Autodesk Inventor part; units mm, degrees
ref_plane "YZ Plane" through (0, 0, 0) normal (1, 0, 0) x (0, 1, 0)
ref_plane "XZ Plane" through (0, 0, 0) normal (0, 1, 0) x (-1, 0, 0)
ref_plane "XY Plane" through (0, 0, 0) normal (0, 0, 1) x (1, 0, 0)
sketch "Sketch1" plane through (0, 0, 0) normal (0, 0, 1) x (1, 0, 0)
  circle A0 centre (0, 0) radius 10.1
  circle A1 centre (0, 0) radius 25
  circle A2 centre (0, 0) radius 17.5 construction
  circle A3 centre (0, 17.5) radius 3
  circle A4 centre (-17.5, 0) radius 3
  circle A5 centre (0, -17.5) radius 3
  circle A6 centre (17.5, 0) radius 3
  line L0 (0, 0) -> (0, 17.5)
  line L1 (0, 0) -> (17.5, 0) construction
  dimension "d0" = 20.2
  dimension "d1" = 50
  dimension "d2" = 35
  dimension "d3" = 6
  dimension "d6" = 360
  dimension "d8" = 90
extrude "Extrusion1" add sketch "Sketch1" along normal blind 5
properties part number "JTW20" material "Brass, Soft Yellow"
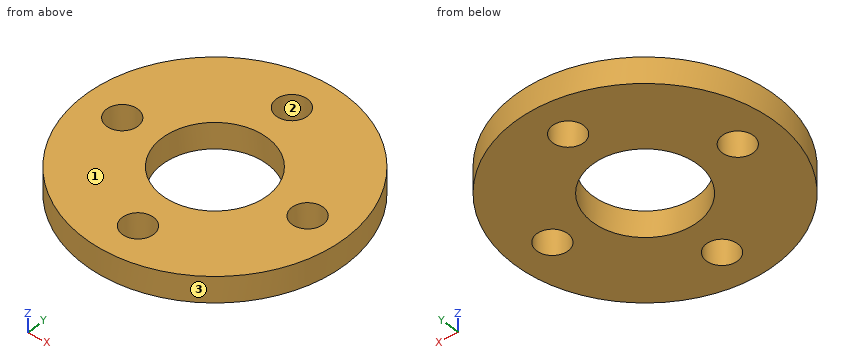
Verification items for the finished model (mm, model axes). Face numbers are marked on the shaded views. Coordinates: 2 decimals unless noted, no trailing zeros. Order: outer loops, then holes, each group sorted by start corner. A loop starts at its lowest first (then second) coordinate and runs counter-clockwise, first axis right, second up. Notation, with made-up numbers: M 16.5,-33 L 73.5,-33 A23 ccw 73.5,-9 Z; hole C -8.75,54 d10. An arc over 180 degrees is marked long. One line per item, written item: value. Start each with the question number.
Item 1: Gauge pin test, flat ends, axial feed: pin 1 (8 mm diameter, centred on x = 0, y = -17.5, fed in from +Z); pin 2 (2 mm diameter, centred on x = 14.5, z = 3.5, fed in from +Y). Record the tip position at first contact, or that the pin passes through.
Item 2: Mould release check, pull along X, two halves, no side actions. Record for the marked faces 1, 2 and 3: released by +X, released by -X, zero draft, split by the parting line, or undercut.
Item 3: Scan lines: probe 1 along Y at (x, z) = (0, 3.9); probe 2 along X at (y, z) = (-2, 2.1); probe 3 along Y at (x, z) = (17.5, 2.6). Record each from-to range of solid material in increasing order.
Item 4: Sectioned sample at A-A (x = 0). Enter the section's corners in (y, z).
Item 5: Sectioned sample at D-D (z = 3.15). Enter the section's corners in (x, y), then the cut area to 3 significant figures.
Item 6: Sectioned sample at B-B (y = -4). Enter the section's corners in (x, z), then the cut area to 3 significant figures.
Item 7: Sectioned sample at C-C (x = 18.5). Enter the section's corners in (y, z), then the cut area to 3 significant figures.
Conclusion:
1. pin 1: stops at z = 5
1. pin 2: stops at y = 21.04
2. face 1: zero draft
2. face 2: undercut
2. face 3: split by the parting line
3. probe 1: y = -25 to -20.5, -14.5 to -10.1, 10.1 to 14.5, 20.5 to 25
3. probe 2: x = -24.92 to -19.74, -15.26 to -9.9, 9.9 to 15.26, 19.74 to 24.92
3. probe 3: y = -17.85 to -3, 3 to 17.85
4. outline: M -25,0 L -20.5,0 L -20.5,5 L -25,5 Z; M -14.5,0 L -10.1,0 L -10.1,5 L -14.5,5 Z; M 10.1,0 L 14.5,0 L 14.5,5 L 10.1,5 Z; M 20.5,0 L 25,0 L 25,5 L 20.5,5 Z
5. outline: C 0,0 d50; hole C -17.5,0 d6; hole C 0,0 d20.2; hole C 0,-17.5 d6; hole C 0,17.5 d6; hole C 17.5,0 d6
5. area: 1,530 mm^2
6. outline: M -24.68,0 L -9.27,0 L -9.27,5 L -24.68,5 Z; M 9.27,0 L 24.68,0 L 24.68,5 L 9.27,5 Z
6. area: 154 mm^2
7. outline: M -16.82,0 L -2.83,0 L -2.83,5 L -16.82,5 Z; M 2.83,0 L 16.82,0 L 16.82,5 L 2.83,5 Z
7. area: 140 mm^2
